```python
from build123d import *

# Parameters (mm, degrees)
CUT_EXTRUDE1_DEPTH  = 2
CUT_EXTRUDE1_DRAFT  = -12
SKETCH3_R           = 2
BOSS_EXTRUDE1_DEPTH = 20


with BuildPart() as part:
    # Sketch1 → Revolve2 (revolve)
    with BuildSketch(Plane(origin=(0, 0, 0), x_dir=(1, 0, 0), z_dir=(0, 1, 0))):
        with BuildLine():
            Line((0, 0), (0, 2))
            Line((0, 2), (2.298285661, 2))
            ThreePointArc((2.298285661, 2), (2.441964308, 1.978911731), (2.57352322, 1.917425786))
            ThreePointArc((2.57352322, 1.917425786), (3.174697589, 1.044998208), (3, 0))
            Line((3, 0), (0, 0))
        make_face()
    revolve(axis=Axis((0, 0, -0.65925001), (0, 0, -1)))


with BuildPart() as cut_extrude1_tool:
    # Sketch2 → Cut-Extrude1 (with draft: the straight prism first)
    with BuildSketch(Plane(origin=(0, 0, -2), x_dir=(-1, 0, 0), z_dir=(0, 0, -1))):
        Polygon((0.5, -0.5), (2, -0.5), (2, 0.5), (0.5, 0.5), (0.5, 2), (-0.5, 2), (-0.5, 0.5), (-2, 0.5), (-2, -0.5), (-0.5, -0.5), (-0.5, -2), (0.5, -2), align=None)
    extrude(amount=-CUT_EXTRUDE1_DEPTH)
    # Cut-Extrude1: the draft: its side faces are tilted about the plane it starts from
    cut_extrude1_sides = [cut_extrude1_tool.faces().sort_by_distance(p)[0] for p in [
        (-1.25, -0.5, -1),
        (-2, 0, -1),
        (-1.25, 0.5, -1),
        (-0.5, 1.25, -1),
        (0, 2, -1),
        (0.5, 1.25, -1),
        (1.25, 0.5, -1),
        (2, 0, -1),
        (1.25, -0.5, -1),
        (0.5, -1.25, -1),
        (0, -2, -1),
        (-0.5, -1.25, -1),
    ]]
    draft(cut_extrude1_sides, Plane(origin=(0, 0, -2), x_dir=(-1, 0, 0), z_dir=(0, 0, -1)), CUT_EXTRUDE1_DRAFT)


with BuildPart() as part_1:
    add(part.part)

    # Cut-Extrude1: cut by cut_extrude1_tool
    add(cut_extrude1_tool.part, mode=Mode.SUBTRACT)

    # Sketch3 → Boss-Extrude1 (add)
    with BuildSketch(Plane.XY):
        with Locations((0.013589602, -0.013589602)):
            Circle(SKETCH3_R)
    extrude(amount=BOSS_EXTRUDE1_DEPTH)


solid = part_1.part
```
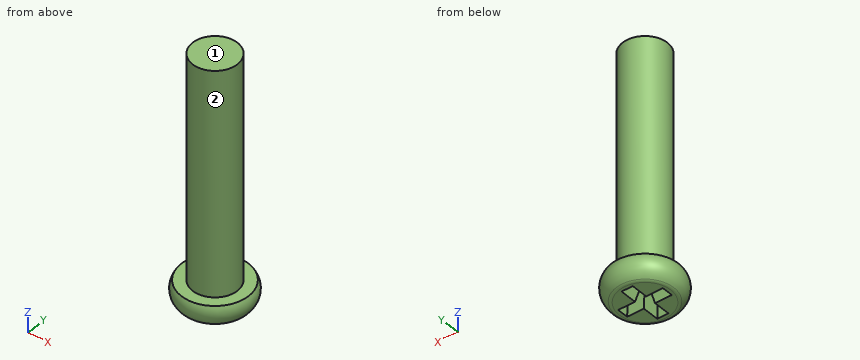
Model file for the job. Use its own axes, mm. Face numbers are marked on the shaded views. A direction names the side the tool comes from. Round coordinates to 2 decimals unless told otherwise and drop trailing zeros. Order: outer loops, then holes, each group sorted by start corner. A loop starts at its lowest first (then second) coordinate and runs counter-clockwise, first axis right, second up. Notation, with made-up numbers: M 51,-18.75 L 98,-18.75 A15 cw 98,-5.75 Z; hole C 15.5,16.25 d9. An arc over 180 degrees is marked long. Use CSV: the item, a comma, the result in double quotes.
Item 1: Saw through at A-A (z = -0.25). List the corners of the cut face in (x, y), plus the area to 3 significant figures.
Worked answers:
outline,"C 0,0 d6.24; hole M -1.63,-0.13 L -0.13,-0.13 L -0.13,-1.63 L 0.13,-1.63 L 0.13,-0.13 L 1.63,-0.13 L 1.63,0.13 L 0.13,0.13 L 0.13,1.63 L -0.13,1.63 L -0.13,0.13 L -1.63,0.13 Z"
area,"29.0 mm²"
Item 2: Which spindle directions (+Z, -Z, +X, -X, +Y, -Y) get a long thin tool onto all of the face, cutting with end or side? Do the marked faces 1 and 2. Say none if no direction does.
Worked answers:
face 1,"+Z, +X, -X, +Y, -Y"
face 2,"+Z"
Item 3: Saw through at B-B (z = 15.5). List the corners of the cut face in (x, y).
Worked answers:
outline,"C 0.01,-0.01 d4"
Item 4: Pin check, flat tips, straight feed: pin 1 (3 mm diameter, centred on y = -2.5, z = 0.5, fed in from -X); pin 2 (1 mm diameter, centred on x = -1, z = 10, fed in from +Y); pin 3 (3 mm diameter, centred on y = 0, z = 12, fed in from -X). Stop position of each tip, or through.
Worked answers:
pin 1,"x = -2.89"
pin 2,"y = 1.92"
pin 3,"x = -1.99"
Item 5: Probe probe 1 along X at (y, z) = (-0.5, -0.75); probe 2 along Y at (x, z) = (0.5, 6.5); probe 3 along Z at (x, y) = (-0.75, 3). List the from-to ranges inside material, lowest first.
Worked answers:
probe 1,"-3.17 to -0.23, 0.23 to 3.17"
probe 2,"-1.95 to 1.93"
probe 3,"-1.3 to -0.18"
